The figure shows three views and two pictorial views of one solid part (mm, origin at its lowest corner). Answer the questions. A direction names the side the tool comes from. Coordinates: 2 decimals unless noted, no trailing zeros. Write each loop counter-clockwise with the first axis right and the second up, starting at its lowest first coordinate (ties: lowest second). Pieces come first, ordered by that corner, then holes.
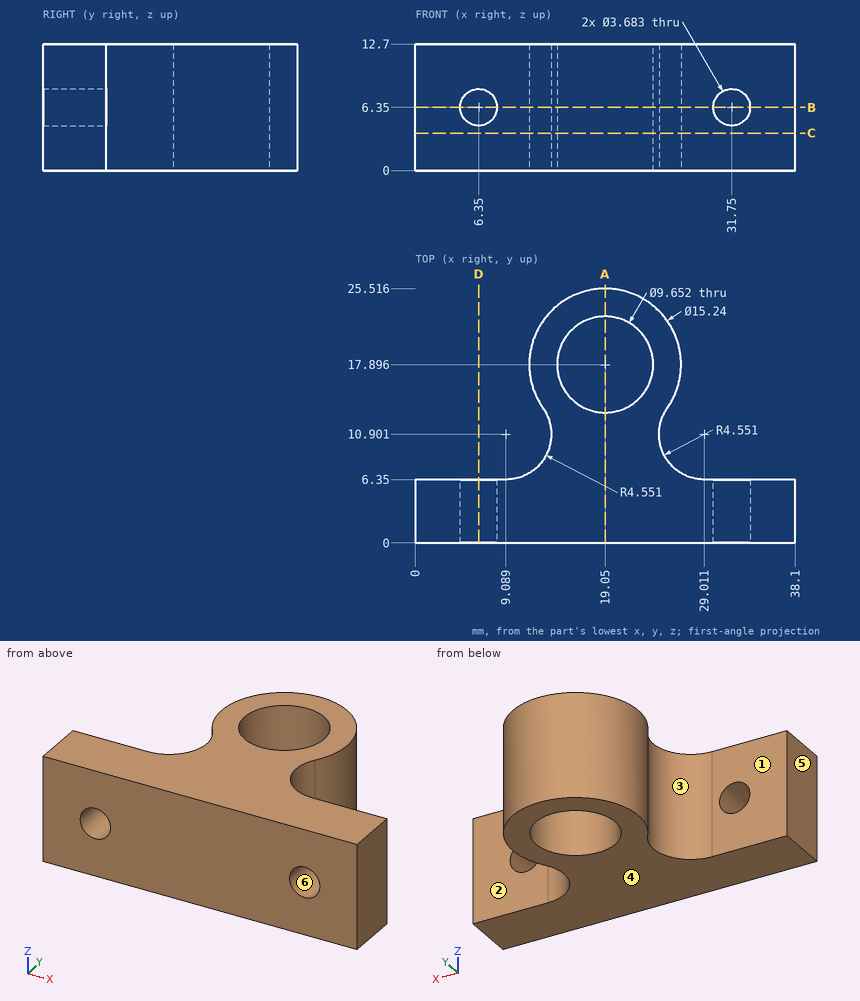
Q1. The part is cut by section A-A, the plane x = 19.05. Write down the section's boundary in (y, z).
Answers below:
outline: (0, 0) - (13.07, 0) - (13.07, 12.7) - (0, 12.7) - close; (22.72, 0) - (25.52, 0) - (25.52, 12.7) - (22.72, 12.7) - close
Q2. The part is cut by section D-D, the plane x = 6.35. Write down the section's boundary in (y, z).
Answers below:
outline: (0, 0) - (6.35, 0) - (6.35, 4.51) - (0, 4.51) - close; (0, 8.19) - (6.35, 8.19) - (6.35, 12.7) - (0, 12.7) - close
Q3. The part is cut by section B-B, the plane z = 6.35. Write down the section's boundary in (x, y), then the cut area to 3 significant figures.
Answers below:
outline: (0, 0) - (4.51, 0) - (4.51, 6.35) - (0, 6.35) - close; (8.19, 0) - (29.91, 0) - (29.91, 6.35) - (29.01, 6.35) arc R4.55 cw to (25.29, 13.52) arc R7.62 ccw (long way) to (12.81, 13.52) arc R4.55 cw to (9.09, 6.35) - (8.19, 6.35) - close; (33.59, 0) - (38.1, 0) - (38.1, 6.35) - (33.59, 6.35) - close; hole circle Ø9.65 at (19.05, 17.9)
area: 364 mm2
Q4. Find the intervals of material crossed by probe 1 along X at (y, z) = (3.5, 6.35); probe 2 along Z at (x, y) = (31.75, 2.75); probe 3 along Y at (x, z) = (19.05, 4.5), in increasing order.
Answers below:
probe 1: x = 0 to 4.51, 8.19 to 29.91, 33.59 to 38.1
probe 2: z = 0 to 4.51, 8.19 to 12.7
probe 3: y = 0 to 13.07, 22.72 to 25.52
Q5. Which of the six approach directions +Z, -Z, +X, -X, +Y, -Y give full straight-line access (tool end or side, diameter ignored) to the marked faces 1, 2 and 3?
Answers below:
face 1: +Z, -Z, -X, +Y
face 2: +Z, -Z, +X, +Y
face 3: +Z, -Z, -X
Q6. The part is cut by section C-C, the plane z = 3.75. Write down the section's boundary in (x, y), then the cut area to 3 significant figures.
Answers below:
outline: (0, 0) - (38.1, 0) - (38.1, 6.35) - (29.01, 6.35) arc R4.55 cw to (25.29, 13.52) arc R7.62 ccw (long way) to (12.81, 13.52) arc R4.55 cw to (9.09, 6.35) - (0, 6.35) - close; hole circle Ø9.65 at (19.05, 17.9)
area: 411 mm2
Q7. Given pin 1 (3 mm diameter, centred on x = 31.75, z = 6.35, fed in from -Y); pin 2 (3 mm diameter, centred on x = 15, y = 11, fed in from -Z); pin 3 (1 mm diameter, centred on x = 29.5, z = 3.5, fed in from +Y); pin 4 (2 mm diameter, centred on x = 9.5, z = 4, fed in from +Y), each flat-ended and moving along its own axis, determine where each tip first touches the part or whether it passes through.
Answers below:
pin 1: passes through
pin 2: stops at z = 0
pin 3: stops at y = 6.35
pin 4: stops at y = 6.57
Q8. Determine the mould class of the marked faces 4, 5 and 6 for opening direction X: released by +X, released by -X, zero draft, split by the parting line, or undercut.
Answers below:
face 4: zero draft
face 5: released by -X
face 6: undercut
